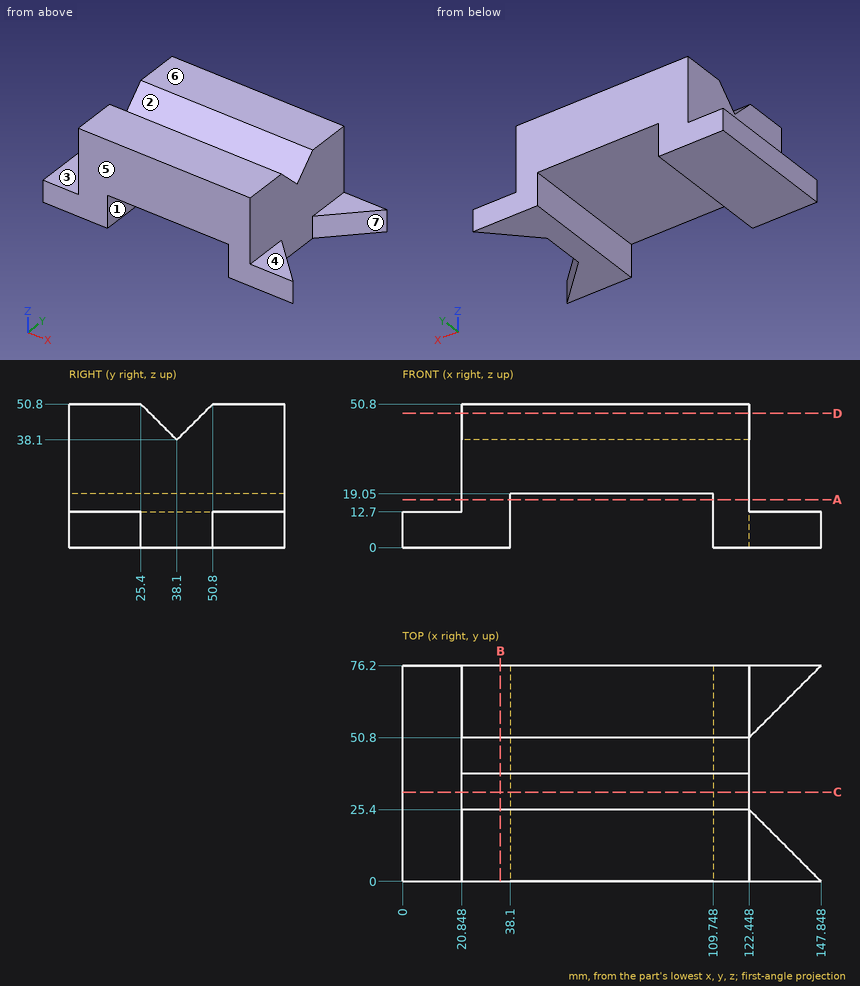
For this review, use the dimensioned drawing (mm, ordinates from the lowest corner) and the shaded views. A direction names the side the tool comes from. Coordinates: 2 decimals unless noted, no trailing zeros. Loops run counter-clockwise (first coordinate to the right, second up) from the corner with the lowest first, then second, coordinate; pieces in that order, holes last.
1. Add section D-D, the plane z = 47.5. Give the boundary of the cut face in (x, y).
2. Add section A-A, the plane z = 17. Give the boundary of the cut face in (x, y).
3. Insertion check: P1, Ø10.5, axis at x = 8.5, y = 32, coming from the +Z side; P2, Ø1, axis at y = 9, z = 17, coming from the +X side; P3, Ø9.5, axis at y = 49.5, z = 12.5, coming from the +X side. Each pin has a flat end and moves straight along its axis. Give the tip position at first contact, or say it passes through.
4. For the marked faces 1, 2, 3 and 4, list the 3-axis set-ups (+Z, -Z, +X, -X, +Y, -Y) from which the entire face can be reached by the end or side of a thin tool; tool diameter is ignored.
5. Add section B-B, the plane x = 34.5. Give the boundary of the cut face in (y, z), then the cut area to 3 significant figures.
6. Add section C-C, the plane y = 31.5. Give the boundary of the cut face in (x, z).
7. Mouldability with a two-part tool opening along Y and no side actions: class the marked faces 5, 6 and 7 as +Y half, -Y half, draft (parallel to the pull), parting line (faces both ways), or undercut.
8. For line 1 (X direction, y = 73, z = 13); line 2 (X direction, y = 32, z = 4.5); line 3 (Y direction, x = 59.5, z = 44.5), list the stretches that pass through material, from the lowest coordinate up.
Result:
1. outline: (20.85, 0) - (122.45, 0) - (122.45, 28.7) - (20.85, 28.7) - close; (20.85, 47.5) - (122.45, 47.5) - (122.45, 76.2) - (20.85, 76.2) - close
2. outline: (20.85, 0) - (38.1, 0) - (38.1, 76.2) - (20.85, 76.2) - close; (109.75, 0) - (122.45, 0) - (122.45, 76.2) - (109.75, 76.2) - close
3. P1: stops at z = 12.7
3. P2: stops at x = 122.45
3. P3: stops at x = 125.9
4. face 1: -Z, +Y, -Y
4. face 2: +Z, +X, -X
4. face 3: +Z, -X, +Y, -Y
4. face 4: +Z, +X, +Y, -Y
5. outline: (0, 0) - (76.2, 0) - (76.2, 50.8) - (50.8, 50.8) - (38.1, 38.1) - (25.4, 50.8) - (0, 50.8) - close
5. area: 3,710 mm2
6. outline: (0, 0) - (38.1, 0) - (38.1, 19.05) - (109.75, 19.05) - (109.75, 0) - (122.45, 0) - (122.45, 44.7) - (20.85, 44.7) - (20.85, 12.7) - (0, 12.7) - close
7. face 5: -Y half
7. face 6: draft
7. face 7: undercut
8. line 1: x = 20.85 to 38.1, 109.75 to 122.45
8. line 2: x = 0 to 38.1, 109.75 to 122.45
8. line 3: y = 0 to 31.7, 44.5 to 76.2
